Here's how the part is built. I have some questions about the finished solid (model axes, mm). A direction names the side the tool comes from. Round coordinates to 2 decimals unless told otherwise and drop trailing zeros. Order: outer loops, then holes, each group sorted by start corner. A loop starts at its lowest first (then second) coordinate and runs counter-clockwise, first axis right, second up. Notation, with made-up numbers: M 79.5,69 L 126.5,69 A28 cw 126.5,88 Z; hole C 17.5,58 d8. An arc over 180 degrees is marked long. Write item = value, one per line. Start each with the question number.
Item 1: I want a section at B-B, the plane y = 2. List the corners of the cut face in (x, z) for me (3 decimals).
Item 2: Please list where these lines run through material, in increasing order: L1, parallel to Z at x = -1.25, y = 2 (3 decimals); L2, parallel to Z at x = 0.5, y = 2 (3 decimals); L3, parallel to Z at x = -4.5, y = 4.25 (3 decimals).
Item 3: We'd pull the mould along Z, two halves only. Please class faces 1 (the face through (7.385, 4.249, -21.028)), 2 (the face through (0, 5, 23)), 3 (the face through (-6.5, 5, 6)): pulls with the +Z half, pulls with the -Z half, needs draft (parallel to the pull), parting line crosses it, or undercut.
Item 4: For faces 4 (the face through (6.5, 5, 6)), 5 (the face through (9.5, 4.9, -20)), 6 (the face through (5, 5, -19)), 7 (the face through (-7.385, 4.249, 20.972)), which set-ups out of +Z, -Z, +X, -X, +Y, -Y let a thin tool reach every point of the face, with its end or its side?
Item 5: I'm going to push flat-ended pins straight in: P1, Ø3, axis at x = 0, z = -7.945, coming from the -Y side; P2, Ø1.5, axis at x = -5.5, z = 2.5, coming from the +Y side; P3, Ø4, axis at x = 5, y = 5, coming from the +Z side; P4, Ø3, axis at y = 4.5, z = -12.5, coming from the +X side. Where does each tip first touch, or does it pass through?
Item 6: I want a section at D-D, the plane x = -5. List the corners of the cut face in (y, z) for me (3 decimals).
Item 7: I want a section at C-C, the plane z = 8. List the corners of the cut face in (x, y) for me, plus the area to 3 significant figures.
Item 8: I want a section at A-A, the plane x = 0. List the corners of the cut face in (y, z) for me (3 decimals).
```python
from build123d import *

# Parameters (mm, degrees)
SKETCH1_W           = 20
SKETCH1_H           = 46
BOSS_EXTRUDE1_DEPTH = 10
SKETCH2_R           = 1
SKETCH2_W           = 13
SKETCH2_H           = 23.3
CUT_EXTRUDE1_DEPTH  = 28
SKETCH3_R           = 2.5
CUT_EXTRUDE2_DEPTH  = 4
CUT_EXTRUDE3_START  = -4
SKETCH4_R           = 2.5
CUT_EXTRUDE3_DEPTH  = 4
SKETCH5_W           = 13.5
SKETCH5_H           = 10
CUT_EXTRUDE4_DEPTH  = 1


with BuildPart() as part:
    # Sketch1 → Boss-Extrude1 (new body)
    with BuildSketch(Plane(origin=(0, 0, 0), x_dir=(1, 0, 0), z_dir=(0, 1, 0))):
        Rectangle(SKETCH1_W, SKETCH1_H)
    extrude(amount=BOSS_EXTRUDE1_DEPTH)

    # Sketch2 → Cut-Extrude1 (cut, through all)
    with BuildSketch(Plane(origin=(0, 10, 0), x_dir=(1, 0, 0), z_dir=(0, 1, 0))):
        with Locations(Location((0, 7.945, 0), (0, 0, 270))):
            Circle(SKETCH2_R)
        with Locations(Location((0, -19.455, 0), (0, 0, 90))):
            Circle(SKETCH2_R)
        with Locations((0, -5.755)):
            Rectangle(SKETCH2_W, SKETCH2_H)
    extrude(amount=-CUT_EXTRUDE1_DEPTH, mode=Mode.SUBTRACT)

    # Sketch3 → Cut-Extrude2 (cut)
    with BuildSketch(Plane(origin=(0, 0, -23), x_dir=(-1, 0, 0), z_dir=(0, 0, -1))):
        with Locations((5, 5)):
            Circle(SKETCH3_R)
        with Locations(Location((-5, 5, 0), (0, 0, 180))):
            Circle(SKETCH3_R)
    extrude(amount=-CUT_EXTRUDE2_DEPTH, mode=Mode.SUBTRACT)

    # Sketch4 → Cut-Extrude3 (cut)
    with BuildSketch(Plane.XY.offset(23).offset(CUT_EXTRUDE3_START)):
        with Locations((5, 5)):
            Circle(SKETCH4_R)
        with Locations(Location((-5, 5, 0), (0, 0, 180))):
            Circle(SKETCH4_R)
    extrude(amount=CUT_EXTRUDE3_DEPTH, mode=Mode.SUBTRACT)

    # Sketch5 → Cut-Extrude4 (cut)
    with BuildSketch(Plane(origin=(10, 0, 0), x_dir=(0, 0, -1), z_dir=(1, 0, 0))):
        with Locations((13.25, 5)):
            Rectangle(SKETCH5_W, SKETCH5_H)
    extrude(amount=-CUT_EXTRUDE4_DEPTH, mode=Mode.SUBTRACT)


solid = part.part
```
Filled in:
q1.outline = M -10,-23 L 10,-23 L 10,-20 L 9,-20 L 9,-6.5 L 10,-6.5 L 10,23 L -10,23 Z; hole M -6.5,-5.895 L 6.5,-5.895 L 6.5,17.405 L -6.5,17.405 Z; hole C 0,-7.945 d2; hole C 0,19.455 d2
q2.L1 = -23 to -5.895, 17.405 to 23
q2.L2 = -23 to -8.811, -7.079 to -5.895, 17.405 to 18.589, 20.321 to 23
q2.L3 = -19 to -5.895, 17.405 to 19
q3.face_1 = needs draft
q3.face_2 = pulls with the +Z half
q3.face_3 = undercut
q4.face_4 = +Y, -Y
q4.face_5 = +X, +Y, -Y
q4.face_6 = -Z
q4.face_7 = +Z
q5.P1 = 0
q5.P2 = through
q5.P3 = 19
q5.P4 = 9
q6.outline = M 0,-23 L 2.5,-23 L 2.5,-19 L 7.5,-19 L 7.5,-23 L 10,-23 L 10,-5.895 L 0,-5.895 Z; M 0,17.405 L 10,17.405 L 10,23 L 7.5,23 L 7.5,19 L 2.5,19 L 2.5,23 L 0,23 Z
q7.outline = M -10,0 L -6.5,0 L -6.5,10 L -10,10 Z; M 6.5,0 L 10,0 L 10,10 L 6.5,10 Z
q7.area = 70.0 mm^2
q8.outline = M 0,-23 L 10,-23 L 10,-8.945 L 0,-8.945 Z; M 0,-6.945 L 10,-6.945 L 10,-5.895 L 0,-5.895 Z; M 0,17.405 L 10,17.405 L 10,18.455 L 0,18.455 Z; M 0,20.455 L 10,20.455 L 10,23 L 0,23 Z
